The listing builds one solid part. Answer for the finished solid, in the listing's coordinates (mm). A direction names the side the tool comes from. Coordinates: 2 decimals unless noted, no trailing zeros. Order: outer loops, then holes, each group sorted by start corner. A loop starts at its lowest first (then second) coordinate and runs counter-clockwise, first axis right, second up.
from build123d import *

# Parameters (mm, degrees)
EXTRU_MINCE1_DEPTH      = 190
ESQUISSE2_R             = 2.5
ENL_V_MAT_EXTRU_1_DEPTH = 199.242276016


with BuildPart() as part:
    # Esquisse1 → Extru.-Mince1 (new body)
    with BuildSketch(Plane.XY):
        Polygon((0, 40), (0, 0), (40, 0), (40, 1.5), (1.5, 1.5), (1.5, 40), align=None)
    extrude(amount=EXTRU_MINCE1_DEPTH)

    # Esquisse2 → Enlèv. mat.-Extru.1 (cut, through all)
    with BuildSketch(Plane.ZY):
        with Locations(Location((57, 20, 0), (0, 0, 270))):
            Circle(ESQUISSE2_R)
        with Locations(Location((133, 20, 0), (0, 0, 270))):
            Circle(ESQUISSE2_R)
    extrude(amount=-ENL_V_MAT_EXTRU_1_DEPTH, mode=Mode.SUBTRACT)


solid = part.part
(1) Find section A-A on z = 57. Determine the outline of the cut face in (x, y), then the cut area to 3 significant figures.
(2) Find the intervals of material crossed by probe 1 along Z at (x, y) = (1.25, 20); probe 2 along Y at (x, z) = (1.05, 133); probe 3 along X at (y, z) = (3, 77.5), in increasing order.
(3) Find section B-B on y = 20. Determine the outline of the cut face in (x, z).
(4) The mould has two halves that part along Y. Classify faces 3 (the flat face through (1.5, 20, 94)), 4 (the flat face through (20, 0, 94)), 5 (the cylindrical face through (0.7, 22.5, 57.1)): pulls with the +Y half, pulls with the -Y half, needs draft (parallel to the pull), parting line crosses it, or undercut.
(5) A tool of negligible diameter and unlimited length cuts with its end or side. For faces 1 (the flat face through (21, 1.5, 94)), 2 (the flat face through (1, 11, 0)), from which of +Z, -Z, +X, -X, +Y, -Y can it reach the whole face along a straight path? Write none if from no direction.
(6) Find section C-C on x = 4.5. Determine the outline of the cut face in (y, z), then the cut area to 3 significant figures.
(7) Given pin 1 Ø3 at (x, z) = (10.5, 39) entering from +Y; pin 2 Ø6.5 at (y, z) = (20, 133) entering from +X; pin 3 Ø4 at (y, z) = (20, 57) entering from +X, each flat-ended and moving along its own axis, determine where each tip first touches the part or whether it passes through.
Resolved:
1. outline: (0, 0) - (40, 0) - (40, 1.5) - (1.5, 1.5) - (1.5, 17.5) - (0, 17.5) - close; (0, 22.5) - (1.5, 22.5) - (1.5, 40) - (0, 40) - close
1. area: 110 mm2
2. probe 1: z = 0 to 54.5, 59.5 to 130.5, 135.5 to 190
2. probe 2: y = 0 to 17.5, 22.5 to 40
2. probe 3: x = 0 to 1.5
3. outline: (0, 0) - (1.5, 0) - (1.5, 54.5) - (0, 54.5) - close; (0, 59.5) - (1.5, 59.5) - (1.5, 130.5) - (0, 130.5) - close; (0, 135.5) - (1.5, 135.5) - (1.5, 190) - (0, 190) - close
4. face 3: needs draft
4. face 4: pulls with the -Y half
4. face 5: undercut
5. face 1: +Z, -Z, +X, +Y
5. face 2: -Z, +X, -X, +Y, -Y
6. outline: (0, 0) - (1.5, 0) - (1.5, 190) - (0, 190) - close
6. area: 285 mm2
7. pin 1: stops at y = 1.5
7. pin 2: stops at x = 1.5
7. pin 3: passes through
